from build123d import *
from OCP.BRepFilletAPI import BRepFilletAPI_MakeFillet

# Parameters (mm, degrees)
SKETCH_1_R          = 2.6
SKETCH_1_W          = 72
SKETCH_1_H          = 17
EXTRUDE_1_DEPTH     = 3
FILLET_1_R1         = 0.2
FILLET_1_R2         = 2
SKETCH_2_R          = 1.6
CUT_EXTRUDE_1_DEPTH = 10
CUT_EXTRUDE_4_DEPTH = 3
SKETCH_8_R          = 1.6
CUT_EXTRUDE_5_DEPTH = 3
FILLET_2_R          = 2
SKETCH_10_R         = 1.6
CUT_EXTRUDE_6_DEPTH = 10


with BuildPart() as part:
    # Sketch 1 → Extrude 1 (new body)
    # profile 1 of 2: a face of its own
    with BuildSketch(Plane.XY):
        with BuildLine():
            Line((36, 0), (-36, 0))
            Line((-36, 0), (-36, -8.333333333))
            ThreePointArc((-36, -8.333333333), (-35.292893219, -8.626226552), (-35, -9.333333333))
            Line((-35, -9.333333333), (-34, -9.333333333))
            ThreePointArc((-34, -9.333333333), (-33, -8.333333333), (-32, -9.333333333))
            ThreePointArc((-32, -9.333333333), (-32.292893219, -10.040440115), (-33, -10.333333333))
            Line((-33, -10.333333333), (-33, -24.333333333))
            ThreePointArc((-33, -24.333333333), (-32.292893219, -24.626226552), (-32, -25.333333333))
            ThreePointArc((-32, -25.333333333), (-33, -26.333333333), (-34, -25.333333333))
            Line((-34, -25.333333333), (-35, -25.333333333))
            ThreePointArc((-35, -25.333333333), (-35.292893219, -26.040440115), (-36, -26.333333333))
            Line((-36, -26.333333333), (-36, -33.666666667))
            ThreePointArc((-36, -33.666666667), (-35.292893219, -33.959559885), (-35, -34.666666667))
            Line((-35, -34.666666667), (-34, -34.666666667))
            ThreePointArc((-34, -34.666666667), (-33, -33.666666667), (-32, -34.666666667))
            ThreePointArc((-32, -34.666666667), (-32.292893219, -35.373773448), (-33, -35.666666667))
            Line((-33, -35.666666667), (-33, -49.666666667))
            ThreePointArc((-33, -49.666666667), (-32.292893219, -49.959559885), (-32, -50.666666667))
            ThreePointArc((-32, -50.666666667), (-33, -51.666666667), (-34, -50.666666667))
            Line((-34, -50.666666667), (-35, -50.666666667))
            ThreePointArc((-35, -50.666666667), (-35.292893219, -51.373773448), (-36, -51.666666667))
            Line((-36, -51.666666667), (-36, -60))
            Line((-36, -60), (36, -60))
            Line((36, -60), (36, -51.666666667))
            ThreePointArc((36, -51.666666667), (35.292893219, -51.373773448), (35, -50.666666667))
            Line((35, -50.666666667), (34, -50.666666667))
            ThreePointArc((34, -50.666666667), (32.292893219, -51.373773448), (33, -49.666666667))
            Line((33, -49.666666667), (33, -35.666666667))
            ThreePointArc((33, -35.666666667), (32.292893219, -33.959559885), (34, -34.666666667))
            Line((34, -34.666666667), (35, -34.666666667))
            ThreePointArc((35, -34.666666667), (35.292893219, -33.959559885), (36, -33.666666667))
            Line((36, -33.666666667), (36, -26.333333333))
            ThreePointArc((36, -26.333333333), (35.292893219, -26.040440115), (35, -25.333333333))
            Line((35, -25.333333333), (34, -25.333333333))
            ThreePointArc((34, -25.333333333), (32.292893219, -26.040440115), (33, -24.333333333))
            Line((33, -24.333333333), (33, -10.333333333))
            ThreePointArc((33, -10.333333333), (32.292893219, -8.626226552), (34, -9.333333333))
            Line((34, -9.333333333), (35, -9.333333333))
            ThreePointArc((35, -9.333333333), (35.292893219, -8.626226552), (36, -8.333333333))
            Line((36, -8.333333333), (36, 0))
        make_face()
        with Locations((-15, -6.5)):
            Circle(SKETCH_1_R, mode=Mode.SUBTRACT)
        with Locations((15, -6.5)):
            Circle(SKETCH_1_R, mode=Mode.SUBTRACT)
    # profile 2 of 2: a face of its own
    with BuildSketch(Plane.XY):
        with Locations((0, -68.5)):
            Rectangle(SKETCH_1_W, SKETCH_1_H)
    extrude(amount=EXTRUDE_1_DEPTH)

    # Fillet 1: one fillet with a radius per group of edges: ONE call of the kernel's fillet builder (fillet() takes one radius for all edges)
    fillet_1_edges_1 = [part.edges().sort_by_distance(p)[0] for p in [
        (-35, -9.333333333, 1.5),
        (-34, -9.333333333, 1.5),
        (33, -10.333333333, 1.5),
        (34, -9.333333333, 1.5),
        (35, -9.333333333, 1.5),
        (36, -8.333333333, 1.5),
        (36, 0, 1.5),
        (-36, 0, 1.5),
        (-36, -8.333333333, 1.5),
        (-33, -10.333333333, 1.5),
        (-33, -24.333333333, 1.5),
        (-34, -25.333333333, 1.5),
        (-35, -25.333333333, 1.5),
        (-36, -26.333333333, 1.5),
        (-36, -33.666666667, 1.5),
        (-35, -34.666666667, 1.5),
        (-34, -34.666666667, 1.5),
        (-33, -35.666666667, 1.5),
        (-33, -49.666666667, 1.5),
        (-34, -50.666666667, 1.5),
        (-35, -50.666666667, 1.5),
        (-36, -51.666666667, 1.5),
        (36, -51.666666667, 1.5),
        (35, -50.666666667, 1.5),
        (34, -50.666666667, 1.5),
        (33, -49.666666667, 1.5),
        (33, -35.666666667, 1.5),
        (34, -34.666666667, 1.5),
        (35, -34.666666667, 1.5),
        (36, -33.666666667, 1.5),
        (36, -26.333333333, 1.5),
        (35, -25.333333333, 1.5),
        (34, -25.333333333, 1.5),
        (33, -24.333333333, 1.5),
    ]]
    fillet_1_edges_2 = [part.edges().sort_by_distance(p)[0] for p in [
        (-36, -77, 1.5),
        (36, -77, 1.5),
    ]]
    fillet_1 = BRepFilletAPI_MakeFillet(part.part.solid().wrapped)
    for e in fillet_1_edges_1:
        fillet_1.Add(FILLET_1_R1, e.wrapped)
    for e in fillet_1_edges_2:
        fillet_1.Add(FILLET_1_R2, e.wrapped)
    add(Compound.cast(fillet_1.Shape()), mode=Mode.REPLACE)

    # Sketch 2 → Cut-Extrude 1 (cut)
    with BuildSketch(Plane.XY.offset(3)):
        with Locations((-23, -20)):
            Circle(SKETCH_2_R)
        with Locations((23, -20)):
            Circle(SKETCH_2_R)
    extrude(amount=-CUT_EXTRUDE_1_DEPTH, mode=Mode.SUBTRACT)

    # Sketch 4 → Cut-Extrude 4 (cut)
    with BuildSketch(Plane.XY.offset(3)):
        Polygon((30.420434699, -62), (-1.373235094, -62), (-1.373235094, -50), (23.858682277, -50), align=None)
    extrude(amount=-CUT_EXTRUDE_4_DEPTH, mode=Mode.SUBTRACT)

    # Sketch 8 → Cut-Extrude 5 (cut)
    with BuildSketch(Plane.XY.offset(3)):
        with Locations((23, -72)):
            Circle(SKETCH_8_R)
        with Locations(Location((-23, -72, 0), (0, 0, 180))):
            Circle(SKETCH_8_R)
    extrude(amount=-CUT_EXTRUDE_5_DEPTH, mode=Mode.SUBTRACT)

    # Fillet 2
    fillet_2_edges = [part.edges().sort_by_distance(p)[0] for p in [
        (23.858682277, -50, 1.5),
        (30.420434699, -62, 1.5),
        (-1.373235094, -62, 1.5),
        (-1.373235094, -50, 1.5),
    ]]
    fillet(fillet_2_edges, radius=FILLET_2_R)

    # Sketch 10 → Cut-Extrude 6 (cut)
    with BuildSketch(Plane.XY.offset(3)):
        with Locations((-12, -30)):
            Circle(SKETCH_10_R)
        with Locations((-12, -40)):
            Circle(SKETCH_10_R)
        with Locations((12, -40)):
            Circle(SKETCH_10_R)
        with Locations((12, -30)):
            Circle(SKETCH_10_R)
    extrude(amount=-CUT_EXTRUDE_6_DEPTH, mode=Mode.SUBTRACT)


solid = part.part
Geometry check sheet. Reference: the model listing, model coordinates, mm. A direction names the side the tool comes from. Round coordinates to 2 decimals unless told otherwise and drop trailing zeros. Loops run counter-clockwise (first coordinate to the right, second up) from the corner with the lowest first, then second, coordinate; pieces in that order, holes last. Notation, with made-up numbers: (-18, 65.25) - (3, 65.25) arc R15 ccw to (3, 90.25) - close; hole circle Ø1 at (75.5, 13). An arc over 180 degrees is marked (long way). One line per question, with ' | ' between items. Start each with the question number.
1. Cross-section at D-D on x = 2. Record the cut outline in (y, z).
2. Scan lines: line 1 (Y direction, x = -12, z = 1); line 2 (X direction, y = -21, z = 2.45); line 3 (Y direction, x = 12, z = 2.4). Record each from-to range of solid material in increasing order. Write a range as [from, to].
3. Cross-section at B-B on y = -72. Record the cut outline in (x, z).
4. Cross-section at A-A on x = -15. Record the cut outline in (y, z).
5. Cross-section at C-C on x = -23. Record the cut outline in (y, z).
6. Tool access check on faces 5 (the face through (-33, -17, 1)), 6 (the face through (33, -17, 1)), 7 (the face through (23.71, -50.29, 1.48)), 8 (the face through (35.43, -76.4, 1.52)), 9 (the face through (36, -4, 1)). Record the directions out of +Z, -Z, +X, -X, +Y, -Y that give a thin tool (end or side, any length) a straight path to the whole face; none if there is none.
7. Depth check by flat-ended pin: pin 1 (0.7 mm diameter, centred on x = 34.5, z = 1, fed in from -Y). Enter the tip coordinate at first touch or a pass-through.
8. Draft check along Y on faces 1 (the face through (1, 0, 1)), 2 (the face through (-1, -38, 3)), 3 (the face through (14, -62, 2)), 4 (the face through (-0.8, -61.4, 1.5)). Enter one of: released by +Y, released by -Y, zero draft, split by the parting line, or undercut.
Taken from the geometry:
1) outline: (-77, 0) - (-62, 0) - (-62, 3) - (-77, 3) - close; (-50, 0) - (0, 0) - (0, 3) - (-50, 3) - close
2) line 1: [-77, -41.6], [-38.4, -31.6], [-28.4, 0] | line 2: [-33, -24.25], [-21.75, 21.75], [24.25, 33] | line 3: [-77, -62], [-50, -41.6], [-38.4, -31.6], [-28.4, 0]
3) outline: (-36, 0) - (-24.6, 0) - (-24.6, 3) - (-36, 3) - close; (-21.4, 0) - (21.4, 0) - (21.4, 3) - (-21.4, 3) - close; (24.6, 0) - (36, 0) - (36, 3) - (24.6, 3) - close
4) outline: (-77, 0) - (-9.1, 0) - (-9.1, 3) - (-77, 3) - close; (-3.9, 0) - (0, 0) - (0, 3) - (-3.9, 3) - close
5) outline: (-77, 0) - (-73.6, 0) - (-73.6, 3) - (-77, 3) - close; (-70.4, 0) - (-21.6, 0) - (-21.6, 3) - (-70.4, 3) - close; (-18.4, 0) - (0, 0) - (0, 3) - (-18.4, 3) - close
6) face 5: +Z, -Z, -X | face 6: +Z, -Z, +X | face 7: +Z, -Z | face 8: +Z, -Z, +X, -Y | face 9: +Z, -Z, +X, +Y, -Y
7) pin 1: y = -76.99
8) face 1: released by +Y | face 2: zero draft | face 3: undercut | face 4: undercut
